Can you work these out from the model? Positions are in its coordinate system, mm. Face numbers are marked on the shaded views. A direction names the side the tool comes from. Round coordinates to 2 decimals unless told otherwise and drop trailing zeros. Loops run counter-clockwise (first coordinate to the right, second up) from the corner with the lowest first, then second, coordinate; pieces in that order, holes last. Notation, with made-up numbers: (46.5, 22.25) -> (54.5, 22.25) arc R23 cw to (54.5, 58.25) -> close; hole circle Ø10 at (-32, -27.5). An arc over 180 degrees is marked (long way). Write each question's results on one line, items separated by ' | '.
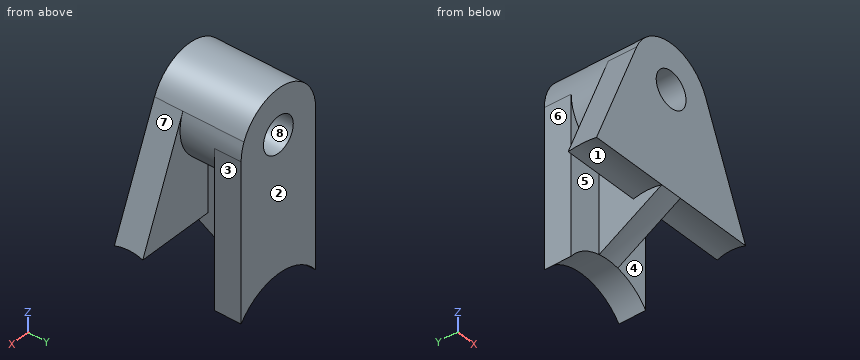
from build123d import *

# Parameters (mm, degrees)
BOSS_EXTRUDE1_DEPTH = 6.35
SKETCH1_3_R         = 10
SKETCH1_3_R_2       = 4
BOSS_EXTRUDE2_DEPTH = 20
SKETCH2_R           = 12.5
CUT_EXTRUDE1_DEPTH  = 55.990908339
BOSS_EXTRUDE3_START = -6
BOSS_EXTRUDE3_DEPTH = 6


with BuildPart() as part:
    # Sketch1 → Boss-Extrude1 (new body)
    with BuildSketch(Plane(origin=(0, 0, 0), x_dir=(1, 0, 0), z_dir=(0, 1, 0))):
        with BuildLine():
            Line((40, 0), (0, 0))
            Line((0, 0), (10.769230769, -25.846153846))
            ThreePointArc((10.769230769, -25.846153846), (18.038838649, -12.194193243), (30, -22))
            ThreePointArc((30, -22), (29.805806757, -23.961161351), (29.230769231, -25.846153846))
            Line((29.230769231, -25.846153846), (40, 0))
        make_face()
    extrude(amount=BOSS_EXTRUDE1_DEPTH)

    # Sketch1_3 → Boss-Extrude2 (add)
    with BuildSketch(Plane(origin=(0, 0, 0), x_dir=(1, 0, 0), z_dir=(0, 1, 0))):
        with Locations(Location((20, -22, 0), (0, 0, 337.380135052))):
            Circle(SKETCH1_3_R)
        with Locations(Location((20, -22, 0), (0, 0, 270))):
            Circle(SKETCH1_3_R_2, mode=Mode.SUBTRACT)
    extrude(amount=BOSS_EXTRUDE2_DEPTH)

    # Sketch2 → Cut-Extrude1 (cut, through all)
    with BuildSketch(Plane(origin=(0, 0, 0), x_dir=(0, 0, -1), z_dir=(1, 0, 0))):
        with Locations((12.090052729, 3.175)):
            Circle(SKETCH2_R)
    extrude(amount=CUT_EXTRUDE1_DEPTH, mode=Mode.SUBTRACT)

    # Sketch3 → Boss-Extrude3 (add)
    with BuildSketch(Plane(origin=(0, 20, 0), x_dir=(1, 0, 0), z_dir=(0, 1, 0)).offset(BOSS_EXTRUDE3_START)):
        with BuildLine():
            Line((10, 13), (10, -22))
            ThreePointArc((10, -22), (20, -12), (30, -22))
            Line((30, -22), (30, 13))
            ThreePointArc((30, 13), (20, 8), (10, 13))
        make_face()
    extrude(amount=BOSS_EXTRUDE3_DEPTH)

    # Sketch5 for Loft1 → Loft1 section 0
    with BuildSketch(Plane.XZ):
        with BuildLine():
            Line((22.5, 0), (17.5, 0))
            Line((17.5, 0), (17.5, 12.317541634))
            # circular arc as an exact rational Bezier (weights 1, cos(half-angle), 1)
            Bezier((17.5, 12.317541634), (20, 11.67204441), (22.5, 12.317541634), weights=[1, 0.968245837, 1])
            Line((22.5, 12.317541634), (22.5, 0))
        make_face()
    # Sketch4 for Loft1 → Loft1 section 1
    with BuildSketch(Plane.XZ.offset(-14)):
        with BuildLine():
            Line((17.5, -8.252551286), (17.5, 12.317541634))
            Bezier((17.5, 12.317541634), (20, 11.67204441), (22.5, 12.317541634), weights=[1, 0.968245837, 1])
            Line((22.5, 12.317541634), (22.5, -8.252551286))
            Bezier((22.5, -8.252551286), (20, -7.742240923), (17.5, -8.252551286), weights=[1, 0.979795897, 1])
        make_face()
    loft()


solid = part.part
1. If we section it at D-D (z = 16.5): List the corners of the cut face in (x, y) for me (3 decimals).
Final values:
outline: (6.875, 0) -> (33.125, 0) -> (33.125, 6.35) -> (28.352, 6.35) -> (28.352, 14) -> (30, 14) -> (30, 20) -> (10, 20) -> (10, 14) -> (11.648, 14) -> (11.648, 6.35) -> (6.875, 6.35) -> close
2. We'd pull the mould along X, two halves only. Please class the marked faces 5, 6, 7 and 8: pulls with the +X half, pulls with the -X half, needs draft (parallel to the pull), parting line crosses it, or undercut.
Final values:
face 5: needs draft | face 6: pulls with the -X half | face 7: pulls with the +X half | face 8: undercut
3. Will these pins go through, and if not, where does the flat tip stop? pin 1 (6 mm diameter, centred on x = 30.5, y = 6.5, fed in from -Z); pin 2 (4 mm diameter, centred on x = 22.5, y = 18, fed in from +Z); pin 3 (1 mm diameter, centred on x = 33, z = 9.5, fed in from +Y).
Final values:
pin 1: z = 0 | pin 2: z = 31.99 | pin 3: y = 6.35
4. Please list where these lines run through material, in increasing order: line 1 (X direction, y = 13.25, z = 22); line 2 (Y direction, x = 8.5, z = 2.5); line 3 (X direction, y = 4.25, z = 25). Write a range as from..to.
Final values:
line 1: 10..16, 24..30 | line 2: 0..6.35 | line 3: 10.42..17.35, 22.65..29.58
5. If we section it at C-C (x = 26.5): List the corners of the cut face in (y, z) for me (3 decimals).
Final values:
outline: (0, 0) arc R12.5 cw to (6.35, 0) -> (6.35, 14.401) -> (14, 14.401) -> (14, -9.823) -> (20, -9.823) -> (20, 29.599) -> (0, 29.599) -> close
6. If we section it at B-B (z = -9): List the corners of the cut face in (x, y) for me.
Final values:
outline: (10, 14) -> (15.1, 14) -> (15.1, 20) -> (10, 20) -> close; (24.9, 14) -> (30, 14) -> (30, 20) -> (24.9, 20) -> close
7. If we section it at A-A (y = 17.5): List the corners of the cut face in (x, z) for me.
Final values:
outline: (10, -13) arc R12.5 cw to (30, -13) -> (30, 22) arc R10 ccw to (10, 22) -> close; hole circle Ø8 at (20, 22)
8. On a 3-axis mill with a long thin cutter (end or side, diameter ignored), from which of +Z, -Z, +X, -X, +Y, -Y can I reach the whole of each face in a straight line? I mean the marked faces 1, 2, 3 and 4. Say none if no direction works.
Final values:
face 1: -Z, -X | face 2: +Z, -Z, +X, -X, +Y | face 3: +Z, -Z, +X, +Y | face 4: -Z, +X
